from build123d import *

# Parameters (mm, degrees)
BOSS_EXTRUDE1_DEPTH         = 224.75
F_11_0_191_DIAMETER_HOLE1_D = 4.8514
M5_CLEARANCE_HOLE2_D        = 5.5
M5_CLEARANCE_HOLE1_D        = 5.5
SKETCH11_R                  = 7.625
CUT_EXTRUDE1_DEPTH          = 244.169042699
FILLET1_R                   = 3.175
FILLET2_R                   = 6.35
CUT_EXTRUDE3_DEPTH          = 244.169042826
FILLET3_R                   = 10


with BuildPart() as part:
    # Sketch1 → Boss-Extrude1 (new, symmetric)
    with BuildSketch(Plane.XY):
        Polygon((42.3291, -38.1), (42.3291, 0), (-42.3291, 0), (-42.3291, -38.1), (-40.1701, -38.1), (-40.1701, -2.159), (40.1701, -2.159), (40.1701, -38.1), align=None)
    extrude(amount=BOSS_EXTRUDE1_DEPTH, both=True)

    # 11 _0.191_ Diameter Hole1 (through all)
    with Locations(Plane(origin=(0, 0, 0), x_dir=(1, 0, 0), z_dir=(0, 1, 0))):
        with Locations((28, 214.75), (-28, 214.75), (0, 214.75)):
            Hole(F_11_0_191_DIAMETER_HOLE1_D / 2)

    # M5 Clearance Hole2 (through all)
    with Locations(Plane(origin=(0, 0, 0), x_dir=(-1, 0, 0), z_dir=(0, 1, 0))):
        with Locations((0, 192.75), (-20, 204.75), (20, 204.75)):
            Hole(M5_CLEARANCE_HOLE2_D / 2)

    # M5 Clearance Hole1 (through all)
    with Locations(Plane(origin=(-42.3291, 0, 0), x_dir=(0, 0, -1), z_dir=(-1, 0, 0))):
        with Locations((66.8, 29.1), (66.8, 9), (-8.2, 29.1), (-8.2, 9), (-83.2, 29.1), (-83.2, 9)):
            Hole(M5_CLEARANCE_HOLE1_D / 2)

    # Sketch11 → Cut-Extrude1 (cut, through all)
    with BuildSketch(Plane(origin=(-42.3291, 0, 0), x_dir=(0, 0, -1), z_dir=(1, 0, 0))):
        with Locations(Location((-28.2, -19.05, 0), (0, 0, 90))):
            Circle(SKETCH11_R)
        with Locations(Location((11.8, -19.05, 0), (0, 0, 90))):
            Circle(SKETCH11_R)
    extrude(amount=CUT_EXTRUDE1_DEPTH, mode=Mode.SUBTRACT)

    # Fillet1
    fillet1_edges = [part.edges().sort_by_distance(p)[0] for p in [
        (40.1701, -2.159, 0),
        (-40.1701, -2.159, 0),
    ]]
    fillet(fillet1_edges, radius=FILLET1_R)

    # Fillet2
    fillet2_edges = [part.edges().sort_by_distance(p)[0] for p in [
        (-42.3291, 0, 0),
        (42.3291, 0, 0),
    ]]
    fillet(fillet2_edges, radius=FILLET2_R)

    # Sketch13 → Cut-Extrude3 (cut, through all)
    with BuildSketch(Plane.ZY.offset(42.3291)):
        with BuildLine():
            Line((-71.8, -38.1), (-81.91878248, -29.609333353))
            ThreePointArc((-81.91878248, -29.609333353), (-86.430294475, -27.004610688), (-91.560596625, -26.1))
            Line((-91.560596625, -26.1), (-224.75, -26.1))
            Line((-224.75, -26.1), (-224.75, -38.1))
            Line((-224.75, -38.1), (-71.8, -38.1))
        make_face()
        with BuildLine():
            Line((88.2, -38.1), (224.75, -38.1))
            Line((224.75, -38.1), (224.75, -26.1))
            Line((224.75, -26.1), (107.960596625, -26.1))
            ThreePointArc((107.960596625, -26.1), (102.830294475, -27.004610688), (98.31878248, -29.609333353))
            Line((98.31878248, -29.609333353), (88.2, -38.1))
        make_face()
    extrude(amount=-CUT_EXTRUDE3_DEPTH, mode=Mode.SUBTRACT)

    # Fillet3
    fillet3_edges = [part.edges().sort_by_distance(p)[0] for p in [
        (-41.2496, -26.1, -224.75),
        (-41.2496, -38.1, -71.8),
        (41.2496, -38.1, -71.8),
        (41.2496, -26.1, -224.75),
        (-41.2496, -26.1, 224.75),
        (-41.2496, -38.1, 88.2),
        (41.2496, -38.1, 88.2),
        (41.2496, -26.1, 224.75),
    ]]
    fillet(fillet3_edges, radius=FILLET3_R)


solid = part.part
Geometry check sheet. Reference: the model listing, model coordinates, mm. A direction names the side the tool comes from. Give positions to 0.01 mm unless a question says otherwise; leave off trailing zeros. Loops run counter-clockwise (first coordinate to the right, second up) from the corner with the lowest first, then second, coordinate; pieces in that order, holes last.
(1) Section check A-A on z = -11.8. Record the cut outline in (x, y) (3 decimals), then the cut area to 3 significant figures.
From the geometry:
outline: (-42.329, -38.1) - (-40.17, -38.1) - (-40.17, -26.675) - (-42.329, -26.675) - close; (-42.329, -11.425) - (-40.17, -11.425) - (-40.17, -5.334) arc R3.175 cw to (-36.995, -2.159) - (36.995, -2.159) arc R3.175 cw to (40.17, -5.334) - (40.17, -11.425) - (42.329, -11.425) - (42.329, -6.35) arc R6.35 ccw to (35.979, 0) - (-35.979, 0) arc R6.35 ccw to (-42.329, -6.35) - close; (40.17, -38.1) - (42.329, -38.1) - (42.329, -26.675) - (40.17, -26.675) - close
area: 259 mm2
(2) Release check for a two-part mould opening along Y. For faces 3 (the cylindrical face through (41.234, -20.703, 20.756)), 4 (the cylindrical face through (41.26, -23.09, 221.9)), 5 (the cylindrical face through (41.234, -24.67, -6.647)), 6 (the flat face through (-42.329, -18, 3)) record: released by +Y, released by -Y, zero draft, split by the parting line, or undercut.
From the geometry:
face 3: undercut
face 4: released by -Y
face 5: undercut
face 6: zero draft
(3) Section check C-C on x = -13.5. Record the cut outline in (y, z).
From the geometry:
outline: (-2.16, -224.75) - (0, -224.75) - (0, 224.75) - (-2.16, 224.75) - close
(4) Depth check by flat-ended pin: pin 1 Ø5 at (x, z) = (24, -70.5) entering from -Y; pin 2 Ø7 at (y, z) = (-29.1, 8.2) entering from +X; pin 3 Ø1.7 at (x, z) = (41.5, 184.5) entering from -Y. Enter the tip coordinate at first touch or a pass-through.
From the geometry:
pin 1: stops at y = -2.16
pin 2: stops at x = 42.33
pin 3: stops at y = -26.1
(5) Set-up check for faces 1 (the flat face through (40.17, -18, 3)), 2 (the flat face through (42.329, -19, 3)): record each of +Z, -Z, +X, -X, +Y, -Y from which the full face is reachable in a straight line by a thin tool's end or side.
From the geometry:
face 1: +Z, -Z, -Y
face 2: +Z, -Z, +X, +Y, -Y
(6) Thickness scan on L1, parallel to Z at x = -20, y = -0.85; L2, parallel to X at y = -28, z = -44.5; L3, parallel to X at y = -0.85, z = 204.75. Record the ranges inside material, lowest first.
From the geometry:
L1: z = -224.75 to 202, 207.5 to 224.75
L2: x = -42.33 to -40.17, 40.17 to 42.33
L3: x = -39.15 to -22.75, -17.25 to 17.25, 22.75 to 39.15
(7) Section check B-B on z = -119. Record the cut outline in (x, y) (3 decimals).
From the geometry:
outline: (-42.329, -26.1) - (-40.17, -26.1) - (-40.17, -5.334) arc R3.175 cw to (-36.995, -2.159) - (36.995, -2.159) arc R3.175 cw to (40.17, -5.334) - (40.17, -26.1) - (42.329, -26.1) - (42.329, -6.35) arc R6.35 ccw to (35.979, 0) - (-35.979, 0) arc R6.35 ccw to (-42.329, -6.35) - close
